The listing builds one solid part. Answer for the finished solid, in the listing's coordinates (mm). A direction names the side the tool comes from. Coordinates: 2 decimals unless noted, no trailing zeros. Write each loop counter-clockwise with the first axis right and the second up, starting at its lowest first coordinate (ties: lowest second). Pieces come first, ordered by that corner, then holes.
from build123d import *

# Parameters (mm, degrees)
SKETCH_W        = 64
SKETCH_H        = 61
PAD_DEPTH       = 2
SKETCH001_W     = 5
SKETCH001_H     = 5
PAD001_DEPTH    = 4
SKETCH002_R     = 0.9
POCKET_DEPTH    = 4
SKETCH003_W     = 4
SKETCH003_H     = 4
PAD002_DEPTH    = 24
SKETCH004_R     = 0.9
POCKET001_DEPTH = 4
FILLET_R        = 3
FILLET001_R     = 3
FILLET002_R     = 3
FILLET003_R     = 3
FILLET004_R     = 3
FILLET005_R     = 2.9
FILLET006_R     = 3
FILLET007_R     = 3
FILLET008_R     = 3
FILLET009_R     = 3
SKETCH005_W     = 64
SKETCH005_H     = 35.4
PAD003_DEPTH    = 4
SKETCH006_R     = 3
POCKET002_DEPTH = 2
SKETCH007_R     = 1.45
POCKET003_DEPTH = 5


with BuildPart() as part:
    # Sketch → Pad (new body)
    with BuildSketch(Plane.XY):
        Rectangle(SKETCH_W, SKETCH_H)
    extrude(amount=PAD_DEPTH)

    # Sketch001 (on Face6 of Pad) → Pad001 (join)
    with BuildSketch(Plane.XY.offset(2)):
        with Locations((-18, 28)):
            Rectangle(SKETCH001_W, SKETCH001_H)
        with Locations((18, 28)):
            Rectangle(SKETCH001_W, SKETCH001_H)
        with Locations((-18, -28)):
            Rectangle(SKETCH001_W, SKETCH001_H)
        with Locations((18, -28)):
            Rectangle(SKETCH001_W, SKETCH001_H)
    extrude(amount=PAD001_DEPTH)

    # Sketch002 (on Face26 of Pad001) → Pocket (cut)
    with BuildSketch(Plane.XY.offset(6)):
        with Locations((-18, -28)):
            Circle(SKETCH002_R)
        with Locations((18, -28)):
            Circle(SKETCH002_R)
        with Locations((18, 28)):
            Circle(SKETCH002_R)
        with Locations((-18, 28)):
            Circle(SKETCH002_R)
    extrude(amount=-POCKET_DEPTH, mode=Mode.SUBTRACT)

    # Sketch003 (on Face5 of Pocket) → Pad002 (join)
    with BuildSketch(Plane.XY.offset(2)):
        with Locations((-30, 23.5)):
            Rectangle(SKETCH003_W, SKETCH003_H)
        with Locations((-30, -7.5)):
            Rectangle(SKETCH003_W, SKETCH003_H)
        with Locations((26, 23.5)):
            Rectangle(SKETCH003_W, SKETCH003_H)
        with Locations((26, -7.5)):
            Rectangle(SKETCH003_W, SKETCH003_H)
    extrude(amount=PAD002_DEPTH)

    # Sketch004 (on Face42 of Pad002) → Pocket001 (cut)
    with BuildSketch(Plane.XY.offset(26)):
        with Locations((-30, 23.5)):
            Circle(SKETCH004_R)
        with Locations((26, 23.5)):
            Circle(SKETCH004_R)
        with Locations((26, -7.5)):
            Circle(SKETCH004_R)
        with Locations((-30, -7.5)):
            Circle(SKETCH004_R)
    extrude(amount=-POCKET001_DEPTH, mode=Mode.SUBTRACT)

    # Fillet
    fillet_edges = [part.edges().sort_by_distance(p)[0] for p in [
        (-30, 25.5, 2),
    ]]
    fillet(fillet_edges, radius=FILLET_R)

    # Fillet001
    fillet001_edges = [part.edges().sort_by_distance(p)[0] for p in [
        (-30, 21.5, 2),
    ]]
    fillet(fillet001_edges, radius=FILLET001_R)

    # Fillet002
    fillet002_edges = [part.edges().sort_by_distance(p)[0] for p in [
        (-28, 23.5, 2),
    ]]
    fillet(fillet002_edges, radius=FILLET002_R)

    # Fillet003
    fillet003_edges = [part.edges().sort_by_distance(p)[0] for p in [
        (-30, -9.5, 2),
    ]]
    fillet(fillet003_edges, radius=FILLET003_R)

    # Fillet004
    fillet004_edges = [part.edges().sort_by_distance(p)[0] for p in [
        (-30, -5.5, 2),
    ]]
    fillet(fillet004_edges, radius=FILLET004_R)

    # Fillet005
    fillet005_edges = [part.edges().sort_by_distance(p)[0] for p in [
        (-28, -7.5, 2),
    ]]
    fillet(fillet005_edges, radius=FILLET005_R)

    # Fillet006
    fillet006_edges = [part.edges().sort_by_distance(p)[0] for p in [
        (26, 25.5, 2),
    ]]
    fillet(fillet006_edges, radius=FILLET006_R)

    # Fillet007
    fillet007_edges = [part.edges().sort_by_distance(p)[0] for p in [
        (26, 21.5, 2),
    ]]
    fillet(fillet007_edges, radius=FILLET007_R)

    # Fillet008
    fillet008_edges = [part.edges().sort_by_distance(p)[0] for p in [
        (26, -9.5, 2),
    ]]
    fillet(fillet008_edges, radius=FILLET008_R)

    # Fillet009
    fillet009_edges = [part.edges().sort_by_distance(p)[0] for p in [
        (26, -5.5, 2),
    ]]
    fillet(fillet009_edges, radius=FILLET009_R)

    # Sketch005 (on Face20 of Fillet009) → Pad003 (join)
    with BuildSketch(Plane.XZ.offset(30.5)):
        with Locations((0, 17.7)):
            Rectangle(SKETCH005_W, SKETCH005_H)
    extrude(amount=PAD003_DEPTH)

    # Sketch006 (on Face20 of Pad003) → Pocket002 (cut)
    with BuildSketch(Plane(origin=(0, -30.5, 0), x_dir=(-1, 0, 0), z_dir=(0, 1, 0))):
        with Locations((6, 13.4)):
            Circle(SKETCH006_R)
        with Locations((-6, 13.4)):
            Circle(SKETCH006_R)
        with Locations((6, 25.4)):
            Circle(SKETCH006_R)
        with Locations((-6, 25.4)):
            Circle(SKETCH006_R)
    extrude(amount=-POCKET002_DEPTH, mode=Mode.SUBTRACT)

    # Sketch007 (on Face69 of Pocket002) → Pocket003 (cut)
    with BuildSketch(Plane.XZ.offset(34.5)):
        with Locations((-6, 25.4)):
            Circle(SKETCH007_R)
        with Locations((6, 25.4)):
            Circle(SKETCH007_R)
        with Locations((-6, 13.4)):
            Circle(SKETCH007_R)
        with Locations((6, 13.4)):
            Circle(SKETCH007_R)
    extrude(amount=-POCKET003_DEPTH, mode=Mode.SUBTRACT)


solid = part.part
Q1. The part is cut by section B-B, the plane x = -18. Write down the section's boundary in (y, z).
Answers below:
outline: (-34.5, 0) - (30.5, 0) - (30.5, 6) - (28.9, 6) - (28.9, 2) - (27.1, 2) - (27.1, 6) - (25.5, 6) - (25.5, 2) - (-25.5, 2) - (-25.5, 6) - (-27.1, 6) - (-27.1, 2) - (-28.9, 2) - (-28.9, 6) - (-30.5, 6) - (-30.5, 35.4) - (-34.5, 35.4) - close
Q2. Determine the mould class of faces 1 (the face through (26, 24, 22)), 2 (the face through (3.23, -31.49, 24.25)), 3 (the face through (-20.5, 28, 4)) for opening direction Z: released by +Z, released by -Z, zero draft, split by the parting line, or undercut.
Answers below:
face 1: released by +Z
face 2: undercut
face 3: zero draft
Q3. Find the intervals of material crossed by probe 1 along Z at (x, y) = (6, -33.2); probe 2 along Z at (x, y) = (-6, -31.8); probe 3 along Y at (x, z) = (-19.5, 10), in increasing order.
Answers below:
probe 1: z = 0 to 11.95, 14.85 to 23.95, 26.85 to 35.4
probe 2: z = 0 to 10.4, 16.4 to 22.4, 28.4 to 35.4
probe 3: y = -34.5 to -30.5
Q4. Given pin 1 (2 mm diameter, centred on x = 10.5, z = 4.5, fed in from +Y); pin 2 (3 mm diameter, centred on y = 24, z = 12, fed in from +X); pin 3 (8 mm diameter, centred on x = 9.5, y = -19.5, fed in from +Z), each flat-ended and moving along its own axis, determine where each tip first touches the part or whether it passes through.
Answers below:
pin 1: stops at y = -30.5
pin 2: stops at x = 28
pin 3: stops at z = 2
Q5. The part is cut by section D-D, the plane z = 32. Write down the section's boundary in (x, y).
Answers below:
outline: (-32, -34.5) - (32, -34.5) - (32, -30.5) - (-32, -30.5) - close
Q6. Which of the six approach directions +Z, -Z, +X, -X, +Y, -Y give full straight-line access (tool end or side, diameter ignored) to faces 4 (the face through (-18, 25.5, 4)), 5 (the face through (-20.5, -28, 4)), 6 (the face through (20.5, -28, 4)), 7 (the face through (26, -9.5, 15)), 8 (the face through (15.5, 28, 4))?
Answers below:
face 4: +Z
face 5: +Z, -X, +Y
face 6: +Z, +X, +Y
face 7: +Z, +X, -X
face 8: +Z, +Y
Q7. The part is cut by section C-C, the plane x = 26. Write down the section's boundary in (y, z).
Answers below:
outline: (-34.5, 0) - (30.5, 0) - (30.5, 2) - (28.5, 2) arc R3 cw to (25.5, 5) - (25.5, 26) - (24.4, 26) - (24.4, 22) - (22.6, 22) - (22.6, 26) - (21.5, 26) - (21.5, 5) arc R3 cw to (18.5, 2) - (-2.5, 2) arc R3 cw to (-5.5, 5) - (-5.5, 26) - (-6.6, 26) - (-6.6, 22) - (-8.4, 22) - (-8.4, 26) - (-9.5, 26) - (-9.5, 5) arc R3 cw to (-12.5, 2) - (-30.5, 2) - (-30.5, 35.4) - (-34.5, 35.4) - close
Q8. The part is cut by section A-A, the plane y = 23.5. Write down the section's boundary in (x, z).
Answers below:
outline: (-32, 0) - (32, 0) - (32, 2) - (28, 2) - (28, 26) - (26.9, 26) - (26.9, 22) - (25.1, 22) - (25.1, 26) - (24, 26) - (24, 2) - (-25, 2) arc R3 cw to (-28, 5) - (-28, 26) - (-29.1, 26) - (-29.1, 22) - (-30.9, 22) - (-30.9, 26) - (-32, 26) - close
